Could you check a few things on this model? Use its own coordinates, in mm. Give positions to 0.01 mm unless a question says otherwise; leave off trailing zeros. Write each loop counter-clockwise with the first axis right and the second up, starting at its lowest first coordinate (ties: lowest second). Pieces come first, ordered by that corner, then holes. Notation, with made-up numbers: (28, 23.25) - (56, 23.25) arc R13 cw to (56, 27.25) - close; hole circle Ø3 at (70, -31). An arc over 180 degrees is marked (long way). Answer as CSV lines item,"result". Start each with the question number.
Q1. Imagine slicing it at A-A on x = -0.5. List the corners of the cut face in (y, z) for me, and give its area (3 significant figures).
Q2. Imagine slicing it at C-C on z = 0. State how many separate pieces and enclosed holes the cut face has, and give its area (3 significant figures).
Q3. If I drill on line 1 along Y through (x, z) = (-8.9, 0); line 2 along X through (y, z) = (615.5, 0), over which ranges is the centre line in solid material (lowest first)?
Q4. Will this pin go through, and if not, where does the flat tip stop? pin 1 Ø6.5 at (y, z) = (349.25, 0) entering from -X.
Q5. Imagine slicing it at B-B on y = 721. List the corners of the cut face in (x, z) for me, and give its area (3 significant figures).
```python
from build123d import *

# Parameters (mm, degrees)
SKETCH1_W                  = 19.304
SKETCH1_H                  = 19.304
SKETCH1_W_2                = 16.764
SKETCH1_H_2                = 16.764
BOSS_EXTRUDE1_DEPTH        = 1308.1
FILLET1_R                  = 1.27
F_1_0_228_DIAMETER_HOLE1_D = 5.7912


with BuildPart() as part:
    # Sketch1 → Boss-Extrude1 (new body)
    with BuildSketch(Plane(origin=(0, 0, 0), x_dir=(1, 0, 0), z_dir=(0, 1, 0))):
        Rectangle(SKETCH1_W, SKETCH1_H)
        Rectangle(SKETCH1_W_2, SKETCH1_H_2, mode=Mode.SUBTRACT)
    extrude(amount=BOSS_EXTRUDE1_DEPTH)

    # Fillet1
    fillet1_edges = [part.edges().sort_by_distance(p)[0] for p in [
        (-8.382, 654.05, 8.382),
        (8.382, 654.05, 8.382),
        (8.382, 654.05, -8.382),
        (-8.382, 654.05, -8.382),
        (9.652, 654.05, 9.652),
        (-9.652, 654.05, 9.652),
        (-9.652, 654.05, -9.652),
        (9.652, 654.05, -9.652),
    ]]
    fillet(fillet1_edges, radius=FILLET1_R)

    # #1 (0.228) Diameter Hole1 (through all)
    with Locations(Plane(origin=(9.652, 0, 0), x_dir=(0, 0, -1), z_dir=(1, 0, 0))):
        with Locations((0, 44.45), (0, 1263.65), (0, 958.85), (0, 654.05), (0, 349.25)):
            Hole(F_1_0_228_DIAMETER_HOLE1_D / 2)


solid = part.part
```
Conclusion:
1,outline,"(0, -9.65) - (1308.1, -9.65) - (1308.1, -8.38) - (0, -8.38) - close; (0, 8.38) - (1308.1, 8.38) - (1308.1, 9.65) - (0, 9.65) - close"
1,area,"3,320 mm^2"
2,separate pieces,"12"
2,enclosed holes,"0"
2,area,"3,250 mm^2"
3,line 1,"0 to 41.55, 47.35 to 346.35, 352.15 to 651.15, 656.95 to 955.95, 961.75 to 1260.75, 1266.55 to 1308.1"
3,line 2,"-9.65 to -8.38, 8.38 to 9.65"
4,pin 1,"x = -9.65"
5,outline,"(-9.65, -8.38) arc R1.27 ccw to (-8.38, -9.65) - (8.38, -9.65) arc R1.27 ccw to (9.65, -8.38) - (9.65, 8.38) arc R1.27 ccw to (8.38, 9.65) - (-8.38, 9.65) arc R1.27 ccw to (-9.65, 8.38) - close; hole (-8.38, -7.11) arc R1.27 ccw to (-7.11, -8.38) - (7.11, -8.38) arc R1.27 ccw to (8.38, -7.11) - (8.38, 7.11) arc R1.27 ccw to (7.11, 8.38) - (-7.11, 8.38) arc R1.27 ccw to (-8.38, 7.11) - close"
5,area,"91.6 mm^2"
